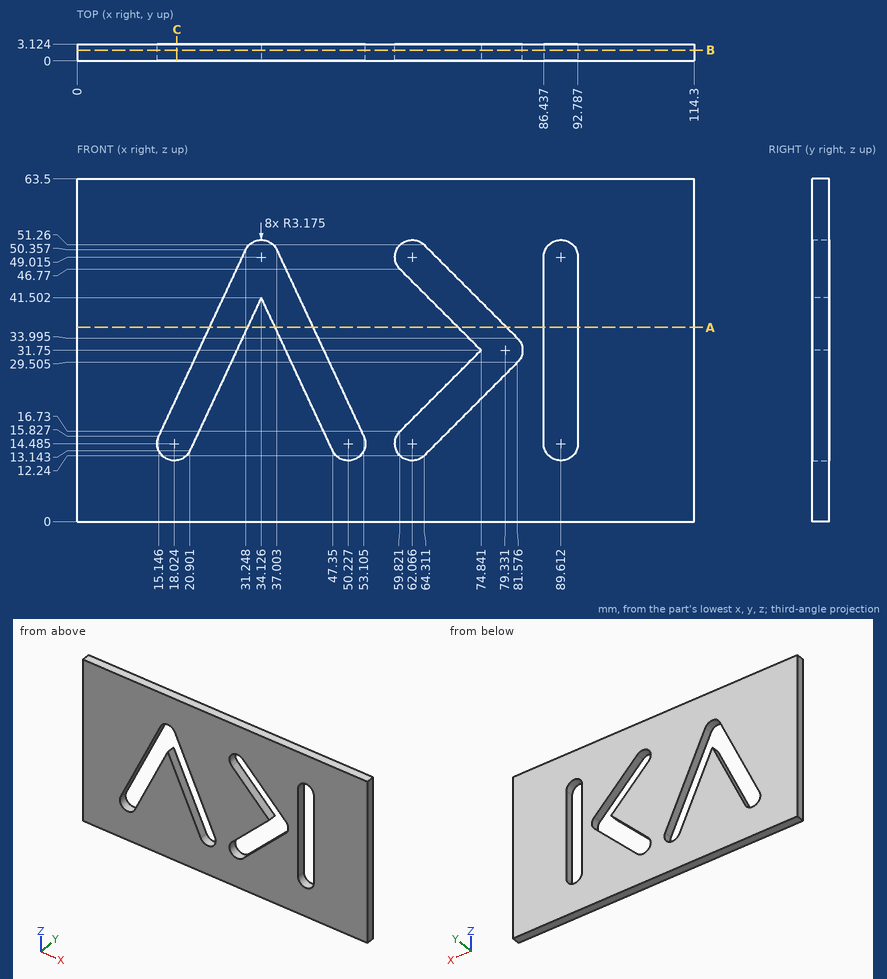
For this review, use the dimensioned drawing (mm, ordinates from the lowest corner) and the shaded views. Round coordinates to 2 decimals unless told otherwise and drop trailing zeros. Write each loop counter-clockwise with the first axis right and the second up, starting at its lowest first coordinate (ties: lowest second). Pieces come first, ordered by that corner, then holes. Notation, with made-up numbers: (44.5, 86) - (96.5, 86) arc R29 ccw to (96.5, 118) - close; hole circle Ø7 at (18.25, -9.75). An arc over 180 degrees is marked (long way). Answer as a JSON object with one key per item and string values.
1. We need section B-B on y = 2. Count the separate pieces of the cut face and the enclosed holes in it, then the cut area to 3 significant figures.
Response values:
{"separate pieces": "1", "enclosed holes": "3", "area": "6,160 mm2"}
2. To check wall thickness, follow line 1 along X through (y, z) = (1.1, 37) (1 decimal); line 2 along X through (y, z) = (2.05, 50.5) (1 decimal); line 3 along X through (y, z) = (0.45, 23.5) (1 decimal). State the ranges of each line that lie inside material, in increasing order.
Response values:
{"line 1": "x = 0 to 25, 32 to 36.2, 43.2 to 69.6, 78.6 to 86.4, 92.8 to 114.3", "line 2": "x = 0 to 31.3, 36.9 to 59.3, 65.1 to 86.8, 92.4 to 114.3", "line 3": "x = 0 to 18.7, 25.7 to 42.5, 49.5 to 66.6, 75.6 to 86.4, 92.8 to 114.3"}
3. We need section A-A on z = 36. Give the boundary of the cut face in (x, y) (1 decimal).
Response values:
{"outline": "(0, 0) - (24.6, 0) - (24.6, 3.1) - (0, 3.1) - close; (31.6, 0) - (36.7, 0) - (36.7, 3.1) - (31.6, 3.1) - close; (43.7, 0) - (70.6, 0) - (70.6, 3.1) - (43.7, 3.1) - close; (79.6, 0) - (86.4, 0) - (86.4, 3.1) - (79.6, 3.1) - close; (92.8, 0) - (114.3, 0) - (114.3, 3.1) - (92.8, 3.1) - close"}
4. We need section C-C on x = 18.5. Give the boundary of the cut face in (y, z) (1 decimal).
Response values:
{"outline": "(0, 0) - (3.1, 0) - (3.1, 11.3) - (0, 11.3) - close; (0, 23) - (3.1, 23) - (3.1, 63.5) - (0, 63.5) - close"}
